Verification items for the finished model (mm, model axes). A direction names the side the tool comes from. Give positions to 0.01 mm unless a question says otherwise; leave off trailing zeros. Loops run counter-clockwise (first coordinate to the right, second up) from the corner with the lowest first, then second, coordinate; pieces in that order, holes last. Notation, with made-up numbers: (54, -21) - (76, -21) arc R10 ccw to (76, -4) - close; hole circle Ø7 at (-35.5, 66.25). An arc over 180 degrees is marked (long way). Answer in a Markdown table with one row per item.
Autodesk Inventor part; units mm, degrees
ref_plane "YZ Plane" through (0, 0, 0) normal (1, 0, 0) x (0, 1, 0)
ref_plane "XZ Plane" through (0, 0, 0) normal (0, 1, 0) x (-1, 0, 0)
ref_plane "XY Plane" through (0, 0, 0) normal (0, 0, 1) x (1, 0, 0)
sketch "Sketch1" plane through (0, 0, 0) normal (0, 0, 1) x (1, 0, 0)
  line L0 (0, 0) -> (50, 0)
  line L1 (50, 0) -> (50, 10)
  line L2 (50, 10) -> (0, 10)
  line L3 (0, 10) -> (0, 0)
  dimension "d0" = 50
  dimension "d1" = 10
extrude "Extrusion1" add sketch "Sketch1" along normal blind 7
sketch "Sketch2" plane through (0, 0, 0) normal (-1, 0, 0) x (0, 0, 1)
  circle A0 centre (6, 5) radius 3.5
  line L0 (7, 10) -> (7, 0)
  point P0 (0, 0)
  point P1 (7, 5)
  dimension "d4" = 7
  dimension "d33" = 1
extrude "Extrusion2" cut sketch "Sketch2" against normal through all
sketch "Sketch3" plane through (0, 0, 0) normal (0, 0, -1) x (-1, 0, 0)
  line L0 (-50, 0) -> (-50, 10)
  line L1 (0, 10) -> (0, 0)
  line L2 (-50, 10) -> (-38, 10)
  line L3 (-38, 10) -> (-38, 16)
  line L4 (-38, 16) -> (-50, 16)
  line L5 (-50, 16) -> (-50, 10)
  line L6 (0, 10) -> (-12, 10)
  line L7 (-12, 10) -> (-12, 16)
  line L8 (-12, 16) -> (0, 16)
  line L9 (0, 16) -> (0, 10)
  line L10 (0, 0) -> (-12, 0)
  line L11 (-12, 0) -> (-12, -6)
  line L12 (-12, -6) -> (0, -6)
  line L13 (0, -6) -> (0, 0)
  line L14 (-50, 0) -> (-38, 0)
  line L15 (-38, 0) -> (-38, -6)
  line L16 (-38, -6) -> (-50, -6)
  line L17 (-50, -6) -> (-50, 0)
  circle A0 centre (-44, 13) radius 1.5
  circle A1 centre (-6, 13) radius 1.5
  circle A2 centre (-6, -3) radius 1.5
  circle A3 centre (-44, -3) radius 1.5
  point P0 (-38, 13)
  point P1 (-12, 13)
  point P2 (-12, -3)
  point P3 (-50, -3)
  point P4 (-44, 16)
  point P5 (-6, 16)
  point P6 (-6, 0)
  point P7 (-44, 0)
  dimension "d15" = 12
  dimension "d16" = 6
  dimension "d17" = 12
  dimension "d18" = 6
  dimension "d19" = 12
  dimension "d20" = 6
  dimension "d21" = 12
  dimension "d22" = 6
  dimension "d23" = 3
  dimension "d24" = 3
  dimension "d25" = 3
  dimension "d26" = 3
extrude "Extrusion3" [suppressed]
sketch "Sketch4" plane through (0, 0, 7) normal (0, 0, 1) x (1, 0, 0)
  line L0 (50, 10) -> (0, 10)
  line L1 (0, 0) -> (50, 0)
  line L2 (10, 10) -> (40, 10)
  line L3 (40, 10) -> (40, 0)
  line L4 (40, 0) -> (10, 0)
  line L5 (10, 0) -> (10, 10)
  point P0 (25, 10)
  dimension "d29" = 30
extrude "Extrusion4" cut sketch "Sketch4" against normal blind 5
sketch "Sketch6" plane through (0, 0, 2) normal (0, 0, 1) x (1, 0, 0)
  line L0 (10, 10) -> (40, 10)
  line L1 (10, 10) -> (40, 10)
  line L2 (40, 10) -> (40, 13)
  line L3 (40, 13) -> (10, 13)
  line L4 (10, 13) -> (10, 10)
  point P0 (0, 0)
  dimension "d41" = 3
extrude "Extrusion6" [suppressed]
sketch "Sketch5" plane through (0, 0, 2) normal (0, 0, 1) x (1, 0, 0)
  circle A0 centre (13, 5) radius 1.5
  circle A1 centre (37, 5) radius 1.5
  line L0 (40, 13) -> (10, 13)
  point P0 (0, 0)
  dimension "d34" = 3
  dimension "d35" = 3
  dimension "d44" = 8
  dimension "d45" = 3
  dimension "d46" = 3
extrude "Extrusion5" cut sketch "Sketch5" against normal blind 10
equation "\"d15\" = d21"
equation "\"d17\" = d21"
equation "\"d19\" = d21"
properties part number "bearing bed2"
Q1. Go/stop test with flat-tipped pins: P1, Ø1, axis at x = 15.5, y = 6, coming from the +Z side; P2, Ø2.5, axis at y = 3, z = 3.5, coming from the -X side; P3, Ø1.5, axis at y = 6, z = 5.5, coming from the +X side. Record where each tip stops, or that it passes through.
Completed:
| item | result |
|---|---|
| P1 | z = 2 |
| P2 | x = 0 |
| P3 | through |
Q2. Tool access check on faces 5 (the face through (44.9, 5.1, 2.5)), 6 (the face through (25, 5, 2)). Record the directions out of +Z, -Z, +X, -X, +Y, -Y that give a thin tool (end or side, any length) a straight path to the whole face; none if there is none.
Completed:
| item | result |
|---|---|
| face 5 | +X, -X |
| face 6 | +Z, +Y, -Y |
Q3. Sectioned sample at A-A (y = 5). Record the cut outline in (x, z), and give its area (3 significant figures).
Completed:
| item | result |
|---|---|
| outline | (0, 0) - (11.5, 0) - (11.5, 2) - (10, 2) - (10, 2.5) - (0, 2.5) - close; (14.5, 0) - (35.5, 0) - (35.5, 2) - (14.5, 2) - close; (38.5, 0) - (50, 0) - (50, 2.5) - (40, 2.5) - (40, 2) - (38.5, 2) - close |
| area | 98.0 mm^2 |
Q4. Sectioned sample at C-C (x = 13). Record the cut outline in (y, z), and give its area (3 significant figures).
Completed:
| item | result |
|---|---|
| outline | (0, 0) - (3.5, 0) - (3.5, 2) - (0, 2) - close; (6.5, 0) - (10, 0) - (10, 2) - (6.5, 2) - close |
| area | 14.0 mm^2 |
Q5. Draft check along Y on faces 1 (the face through (11.5, 5.07, 1.01)), 2 (the face through (40, 5.1, 2.3)), 3 (the face through (25, 0, 1)), 4 (the face through (4.9, 5.1, 2.5)). Enter one of: +Y half, -Y half, draft (parallel to the pull), parting line (faces both ways), or undercut.
Completed:
| item | result |
|---|---|
| face 1 | undercut |
| face 2 | draft |
| face 3 | -Y half |
| face 4 | undercut |
Q6. Sectioned sample at D-D (x = 4). Record the cut outline in (y, z).
Completed:
| item | result |
|---|---|
| outline | (0, 0) - (10, 0) - (10, 7) - (8.35, 7) arc R3.5 cw (long way) to (1.65, 7) - (0, 7) - close |
Q7. Thickness scan on line 1 (X direction, y = 1.75, z = 3); line 2 (Y direction, x = 5.5, z = 6); line 3 (Y direction, x = 37, z = 0.4). Record the ranges inside material, lowest first.
Completed:
| item | result |
|---|---|
| line 1 | 0 to 10, 40 to 50 |
| line 2 | 0 to 1.5, 8.5 to 10 |
| line 3 | 0 to 3.5, 6.5 to 10 |
Q8. Sectioned sample at B-B (z = 6). Record the cut outline in (x, y).
Completed:
| item | result |
|---|---|
| outline | (0, 0) - (10, 0) - (10, 1.5) - (0, 1.5) - close; (0, 8.5) - (10, 8.5) - (10, 10) - (0, 10) - close; (40, 0) - (50, 0) - (50, 1.5) - (40, 1.5) - close; (40, 8.5) - (50, 8.5) - (50, 10) - (40, 10) - close |
